from build123d import *

# Parameters (mm, degrees)
BOSS_EXTRUDE1_DEPTH = 25
SKETCH2_R           = 4
CUT_EXTRUDE1_DEPTH  = 88.229582138
SKETCH3_R           = 1.6
CUT_EXTRUDE2_DEPTH  = 79.755553628
CUT_EXTRUDE3_DEPTH  = 3
FILLET2_R           = 8
CHAMFER2_SIZE       = 10
SKETCH5_W           = 30
SKETCH5_H           = 25
BOSS_EXTRUDE2_DEPTH = 26
SKETCH6_W           = 20.004484435
SKETCH6_H           = 25
BOSS_EXTRUDE3_DEPTH = 44
SKETCH7_W           = 10.4
SKETCH7_H           = 20.4
CUT_EXTRUDE4_DEPTH  = 23
SKETCH9_W           = 20.004484435
SKETCH9_H           = 44
SKETCH9_W_2         = 10.4
SKETCH9_H_2         = 20.4
BOSS_EXTRUDE4_DEPTH = 20
SKETCH10_R          = 2.1
CUT_EXTRUDE6_DEPTH  = 93.726686192
CHAMFER5_SIZE       = 5
SKETCH11_R          = 2
CUT_EXTRUDE7_DEPTH  = 115.564392374
SKETCH12_W          = 20.004484435
SKETCH12_H          = 20
SKETCH12_R          = 2.1
BOSS_EXTRUDE5_DEPTH = 30
SKETCH13_R          = 1.6
CUT_EXTRUDE8_DEPTH  = 107.048283023


with BuildPart() as part:
    # Sketch1 → Boss-Extrude1 (new body)
    with BuildSketch(Plane(origin=(0, 0, 0), x_dir=(1, 0, 0), z_dir=(0, 1, 0))):
        with BuildLine():
            Line((-13.972375691, -8), (-23.972375691, -8))
            Line((-23.972375691, -8), (-23.972375691, -38))
            Line((-23.972375691, -38), (-3.972375691, -38))
            Line((-3.972375691, -38), (-3.972375691, -78))
            Line((-3.972375691, -78), (6.027624309, -78))
            Line((6.027624309, -78), (6.027624309, -38))
            Line((6.027624309, -38), (26.027624309, -38))
            Line((26.027624309, -38), (26.027624309, -8))
            Line((26.027624309, -8), (16.027624309, -8))
            ThreePointArc((16.027624309, -8), (1.027624309, -23), (-13.972375691, -8))
        make_face()
    extrude(amount=BOSS_EXTRUDE1_DEPTH)

    # Sketch2 → Cut-Extrude1 (cut, through all)
    with BuildSketch(Plane.ZY.offset(3.972375691)):
        with Locations((70, 12.5)):
            Circle(SKETCH2_R)
    extrude(amount=-CUT_EXTRUDE1_DEPTH, mode=Mode.SUBTRACT)

    # Sketch3 → Cut-Extrude2 (cut, through all)
    with BuildSketch(Plane(origin=(0, 0, 8), x_dir=(-1, 0, 0), z_dir=(0, 0, -1))):
        with Locations((-21.027624309, 6.5)):
            Circle(SKETCH3_R)
        with Locations((-21.027624309, 18.5)):
            Circle(SKETCH3_R)
        with Locations((18.972375691, 6.5)):
            Circle(SKETCH3_R)
        with Locations((18.972375691, 18.5)):
            Circle(SKETCH3_R)
    extrude(amount=-CUT_EXTRUDE2_DEPTH, mode=Mode.SUBTRACT)

    # Sketch4 → Cut-Extrude3 (cut)
    with BuildSketch(Plane.XY.offset(38)):
        Polygon((24.277624309, 18.5), (22.652624309, 21.314582562), (19.402624309, 21.314582562), (17.777624309, 18.5), (19.402624309, 15.685417438), (22.652624309, 15.685417438), align=None)
        Polygon((24.277624309, 6.5), (22.652624309, 9.314582562), (19.402624309, 9.314582562), (17.777624309, 6.5), (19.402624309, 3.685417438), (22.652624309, 3.685417438), align=None)
        Polygon((-15.722375691, 18.5), (-17.347375691, 21.314582562), (-20.597375691, 21.314582562), (-22.222375691, 18.5), (-20.597375691, 15.685417438), (-17.347375691, 15.685417438), align=None)
        Polygon((-15.722375691, 6.5), (-17.347375691, 9.314582562), (-20.597375691, 9.314582562), (-22.222375691, 6.5), (-20.597375691, 3.685417438), (-17.347375691, 3.685417438), align=None)
    extrude(amount=-CUT_EXTRUDE3_DEPTH, mode=Mode.SUBTRACT)

    # Fillet2
    fillet2_edges = [part.edges().sort_by_distance(p)[0] for p in [
        (1.027624309, 0, 78),
        (1.027624309, 25, 78),
    ]]
    fillet(fillet2_edges, radius=FILLET2_R)

    # Chamfer2
    chamfer2_edges = [part.edges().sort_by_distance(p)[0] for p in [
        (6.027624309, 12.5, 38),
        (-3.972375691, 12.5, 38),
    ]]
    chamfer(chamfer2_edges, length=CHAMFER2_SIZE)

    # Sketch5 → Boss-Extrude2 (add)
    with BuildSketch(Plane.ZY.offset(23.972375691)):
        with Locations((23, 12.5)):
            Rectangle(SKETCH5_W, SKETCH5_H)
    extrude(amount=BOSS_EXTRUDE2_DEPTH)

    # Sketch6 → Boss-Extrude3 (add)
    with BuildSketch(Plane.XY.offset(38)):
        with Locations((-39.970133473, 12.5)):
            Rectangle(SKETCH6_W, SKETCH6_H)
    extrude(amount=BOSS_EXTRUDE3_DEPTH)

    # Sketch7 → Cut-Extrude4 (cut)
    with BuildSketch(Plane.XZ):
        with Locations((-39.970133474, 66)):
            Rectangle(SKETCH7_W, SKETCH7_H)
    extrude(amount=-CUT_EXTRUDE4_DEPTH, mode=Mode.SUBTRACT)

    # Sketch9 → Boss-Extrude4 (add)
    with BuildSketch(Plane.XZ):
        with Locations((-39.970133473, 60)):
            Rectangle(SKETCH9_W, SKETCH9_H)
        with Locations((-39.970133474, 66)):
            Rectangle(SKETCH9_W_2, SKETCH9_H_2, mode=Mode.SUBTRACT)
    extrude(amount=BOSS_EXTRUDE4_DEPTH)

    # Sketch10 → Cut-Extrude6 (cut, through all)
    with BuildSketch(Plane.XY.offset(82)):
        with Locations((-39.970133474, -9.5)):
            Circle(SKETCH10_R)
        with Locations((-39.970133474, 18.5)):
            Circle(SKETCH10_R)
    extrude(amount=-CUT_EXTRUDE6_DEPTH, mode=Mode.SUBTRACT)

    # Chamfer5
    chamfer5_edges = [part.edges().sort_by_distance(p)[0] for p in [
        (-29.967891256, 12.5, 38),
    ]]
    chamfer(chamfer5_edges, length=CHAMFER5_SIZE)

    # Sketch11 → Cut-Extrude7 (cut, through all)
    with BuildSketch(Plane(origin=(26.027624309, 0, 0), x_dir=(0, 0, -1), z_dir=(1, 0, 0))):
        with Locations((-26, 12.5)):
            Circle(SKETCH11_R)
    extrude(amount=-CUT_EXTRUDE7_DEPTH, mode=Mode.SUBTRACT)

    # Sketch12 → Boss-Extrude5 (add)
    with BuildSketch(Plane(origin=(0, 0, 38), x_dir=(-1, 0, 0), z_dir=(0, 0, -1))):
        with Locations((39.970133473, -10)):
            Rectangle(SKETCH12_W, SKETCH12_H)
        with Locations(Location((39.970133474, -9.5, 0), (0, 0, 180))):
            Circle(SKETCH12_R, mode=Mode.SUBTRACT)
    extrude(amount=BOSS_EXTRUDE5_DEPTH)

    # Sketch13 → Cut-Extrude8 (cut, through all)
    with BuildSketch(Plane.XZ.offset(20)):
        with Locations(Location((-33.970133474, 33, 0), (0, 0, 270))):
            Circle(SKETCH13_R)
        with Locations(Location((-45.970133474, 33, 0), (0, 0, 270))):
            Circle(SKETCH13_R)
    extrude(amount=-CUT_EXTRUDE8_DEPTH, mode=Mode.SUBTRACT)


solid = part.part
Geometry: final body of the model. Coordinates: model frame, mm. A direction names the side the tool comes from. Give positions to 0.01 mm unless a question says otherwise; leave off trailing zeros. Loops run counter-clockwise (first coordinate to the right, second up) from the corner with the lowest first, then second, coordinate; pieces in that order, holes last. Notation, with made-up numbers: (-25, 55.25) -> (33, 55.25) arc R29 cw to (33, 94.25) -> close; hole circle Ø7 at (-36, 59.25). An arc over 180 degrees is marked (long way). Put each result on its own line as item: value.
1. Ray query, line 1 along X through (y, z) = (8.5, 69.5); line 2 along X through (y, z) = (14.5, 68); line 3 along X through (y, z) = (16, 33). Return the intervals inside material, ascending. Write a range as [from, to].
Taken from the geometry:
line 1: x = [-49.97, -45.17], [-34.77, -29.97], [-3.97, 6.03]
line 2: x = [-49.97, -45.17], [-34.77, -29.97]
line 3: x = [-49.97, -47.57], [-44.37, -35.57], [-32.37, 26.03]
2. Cut plane D-D (y = -9.5). Return the cut outline in (x, z).
Taken from the geometry:
outline: (-49.97, 8) -> (-42.07, 8) -> (-42.07, 55.8) -> (-45.17, 55.8) -> (-45.17, 76.2) -> (-42.07, 76.2) -> (-42.07, 82) -> (-49.97, 82) -> close; (-37.87, 8) -> (-29.97, 8) -> (-29.97, 82) -> (-37.87, 82) -> (-37.87, 76.2) -> (-34.77, 76.2) -> (-34.77, 55.8) -> (-37.87, 55.8) -> close; hole circle Ø3.2 at (-45.97, 33); hole circle Ø3.2 at (-33.97, 33)
3. Pull-direction query (Y, two-part tool) for faces 6 (the flat face through (-16.524, 19.888, 36.521)), 7 (the flat face through (-27.433, 12.325, 40.465)), 8 (the flat face through (-2, 0, 32)); classes: released by +Y, released by -Y, zero draft, split by the parting line, or undercut.
Taken from the geometry:
face 6: undercut
face 7: zero draft
face 8: released by -Y
4. Cut plane B-B (z = 49). Return the cut outline in (x, y).
Taken from the geometry:
outline: (-49.97, -20) -> (-29.97, -20) -> (-29.97, 25) -> (-49.97, 25) -> close; (-3.97, 0) -> (6.03, 0) -> (6.03, 25) -> (-3.97, 25) -> close; hole circle Ø4.2 at (-39.97, -9.5); hole circle Ø4.2 at (-39.97, 18.5)
5. Pin query (flat end, axial travel): P1, Ø1.7, axis at x = 20.5, y = 17.5, coming from the +Z side; P2, Ø3, axis at x = -7, z = 17, coming from the +Y side; P3, Ø7, axis at y = 12.5, z = 70, coming from the +X side; P4, Ø5, axis at x = 20.5, y = 9, coming from the +Z side. Return the tip coordinate at first contact, or that it passes through.
Taken from the geometry:
P1: stops at z = 35
P2: passes through
P3: stops at x = -29.97
P4: stops at z = 38
6. Cut plane A-A (z = 33). Count the separate pieces of the cut face and the enclosed holes in it, plus the area to 3 significant figures.
Taken from the geometry:
separate pieces: 3
enclosed holes: 6
area: 1,950 mm2
7. Cut plane C-C (z = 25). Return the cut outline in (x, y), plus the area to 3 significant figures.
Taken from the geometry:
outline: (-49.97, -20) -> (-29.97, -20) -> (-29.97, 0) -> (26.03, 0) -> (26.03, 10.77) -> (-49.97, 10.77) -> close; (-49.97, 14.23) -> (26.03, 14.23) -> (26.03, 25) -> (-49.97, 25) -> close; hole circle Ø4.2 at (-39.97, -9.5); hole circle Ø4.2 at (-39.97, 18.5); hole circle Ø3.2 at (-18.97, 6.5); hole circle Ø3.2 at (-18.97, 18.5); hole circle Ø3.2 at (21.03, 6.5); hole circle Ø3.2 at (21.03, 18.5)
area: 1,980 mm2
8. Set-up query: faces 1 (the flat face through (21, 12, 38)), 2 (the cylindrical face through (-41.518, -8.081, 79.141)), 3 (the flat face through (-45.17, 2, 66)), 4 (the cylindrical face through (-35.53, 2.18, 33.35)), 5 (the flat face through (-21.42, 17.11, 36.52)). Return all of +Z, -Z, +X, -X, +Y, -Y with unobstructed straight access to the full face (end or side cutting, diameter ignored); none if empty.
Taken from the geometry:
face 1: +Z, +X, +Y, -Y
face 2: +Z, -Z
face 3: -Y
face 4: +Y, -Y
face 5: +Z
